Check sheet for the modelled part. Datum: model origin and axes. Units: mm. A direction names the side the tool comes from. Give positions to 0.01 mm unless a question says otherwise; leave off trailing zeros. Order: outer loops, then holes, each group sorted by start corner. A loop starts at its lowest first (then second) coordinate and runs counter-clockwise, first axis right, second up.
```python
from build123d import *

# Parameters (mm, degrees)
SKETCH1_R           = 19.5
BOSS_EXTRUDE1_DEPTH = 10
SHELL1_T            = 1.5
SKETCH2_W           = 9
SKETCH2_H           = 6
CUT_EXTRUDE1_DEPTH  = 3


with BuildPart() as part:
    # Sketch1 → Boss-Extrude1 (new body)
    with BuildSketch(Plane(origin=(0, 0, 0), x_dir=(1, 0, 0), z_dir=(0, 1, 0))):
        with Locations(Location((0, 0, 0), (0, 0, 270))):
            Circle(SKETCH1_R)
    extrude(amount=BOSS_EXTRUDE1_DEPTH)

    # Shell1
    shell1_openings = [part.faces().sort_by_distance(p)[0] for p in [
        (0, 10, 0),
    ]]
    offset(amount=SHELL1_T, openings=shell1_openings, kind=Kind.INTERSECTION)

    # Sketch2 → Cut-Extrude1 (cut)
    with BuildSketch(Plane(origin=(-35.117811043, 32.6041754, -20.627520882), x_dir=(-0.9999433956533795, 0, 0.010639806821049314), z_dir=(-0.010639806821049314, 0, -0.9999433956533795))):
        with Locations((-34.896350385, -34.1041754)):
            Rectangle(SKETCH2_W, SKETCH2_H)
    extrude(amount=-CUT_EXTRUDE1_DEPTH, mode=Mode.SUBTRACT)


solid = part.part
```
(1) Material ranges on L1, parallel to X at y = 5.5, z = 0; L2, parallel to Y at x = -12.5, z = 1, recorded low to high.
Response values:
L1: x = -21 to -19.5, 19.5 to 21
L2: y = -1.5 to 0
(2) Cross-section at D-D on x = -5.5. Enter the section's corners in (y, z).
Response values:
outline: (-1.5, -20.27) - (10, -20.27) - (10, -18.71) - (0, -18.71) - (0, 18.71) - (10, 18.71) - (10, 20.27) - (-1.5, 20.27) - close
(3) Release check for a two-part mould opening along Z. For faces 3 (the face through (5.86, 4.93, 18.6)), 4 (the face through (6.31, 4.17, 20.03)), 5 (the face through (-19, 10, 6)) record: released by +Z, released by -Z, zero draft, split by the parting line, or undercut.
Response values:
face 3: undercut
face 4: split by the parting line
face 5: zero draft
(4) Set-up check for faces 1 (the face through (0, 0, 0)), 2 (the face through (0, -1.5, 0)): record each of +Z, -Z, +X, -X, +Y, -Y from which the full face is reachable in a straight line by a thin tool's end or side.
Response values:
face 1: +Y
face 2: +Z, -Z, +X, -X, -Y
(5) Cross-section at A-A on z = 0. Enter the section's corners in (x, y), then the cut area to 3 significant figures.
Response values:
outline: (-21, -1.5) - (21, -1.5) - (21, 10) - (19.5, 10) - (19.5, 0) - (-19.5, 0) - (-19.5, 10) - (-21, 10) - close
area: 93.0 mm2
(6) Gauge pin test, flat ends, axial feed: pin 1 Ø11.5 at (x, z) = (-6.5, -6.5) entering from +Y; pin 2 Ø1 at (x, z) = (-1, -20) entering from -Y; pin 3 Ø3 at (y, z) = (8.5, 16) entering from +X. Record the tip position at first contact, or that the pin passes through.
Response values:
pin 1: stops at y = 0
pin 2: stops at y = 1.5
pin 3: stops at x = 15.19
(7) Cross-section at B-B on x = 0. Enter the section's corners in (y, z), then the cut area to 3 significant figures.
Response values:
outline: (-1.5, -18) - (0, -18) - (0, 19.5) - (10, 19.5) - (10, 21) - (-1.5, 21) - close; (1.5, -21) - (10, -21) - (10, -19.5) - (1.5, -19.5) - close
area: 86.3 mm2
(8) Cross-section at C-C on y = 3. Enter the section's corners in (x, z).
Response values:
outline: circle Ø42 at (0, 0); hole circle Ø39 at (0, 0)
